Here's the drawing with two shaded views (mm, measured from the low corner). I have some questions. A direction names the side the tool comes from. Round coordinates to 2 decimals unless told otherwise and drop trailing zeros. Loops run counter-clockwise (first coordinate to the right, second up) from the corner with the lowest first, then second, coordinate; pieces in that order, holes last.
(1) Will these pins go through, and if not, where does the flat tip stop? pin 1 Ø1.5 at (y, z) = (26, 8.5) entering from -X; pin 2 Ø1.7 at (x, z) = (5, 12) entering from +Y; pin 3 Ø1 at (y, z) = (13.5, 3) entering from +X; pin 4 Ø5 at (x, y) = (16, 26) entering from -Z.
(2) Thinking about a two-plate mould opening in Z: for the marked faces 1, 2, 3 and 4, which applies, released by +Z, released by -Z, zero draft, split by the parting line, or undercut?
(3) Which directions (+Z, -Z, +X, -X, +Y, -Y) give clear straight access to the entire face, cutting with the end or side of a thin tool? Please do the marked faces 5, 6, 7, 8 and 9.
(4) I want a section at C-C on x = 16. Write out the boundary of the cut face in (y, z), plus the area to 3 significant figures.
(5) If I drill on line 1 along Y through (x, z) = (6.25, 8.75); line 2 along Z through (x, y) = (7, 13.25); line 3 along X through (y, z) = (4, 10.75), over which ranges is the centre line in solid material (lowest first)?
(6) I want a section at B-B on x = 5. Write out the boundary of the cut face in (y, z).
(7) I want a section at D-D on y = 26. Write out the boundary of the cut face in (x, z).
(8) I want a section at A-A on z = 4.5. Write out the boundary of the cut face in (x, y).
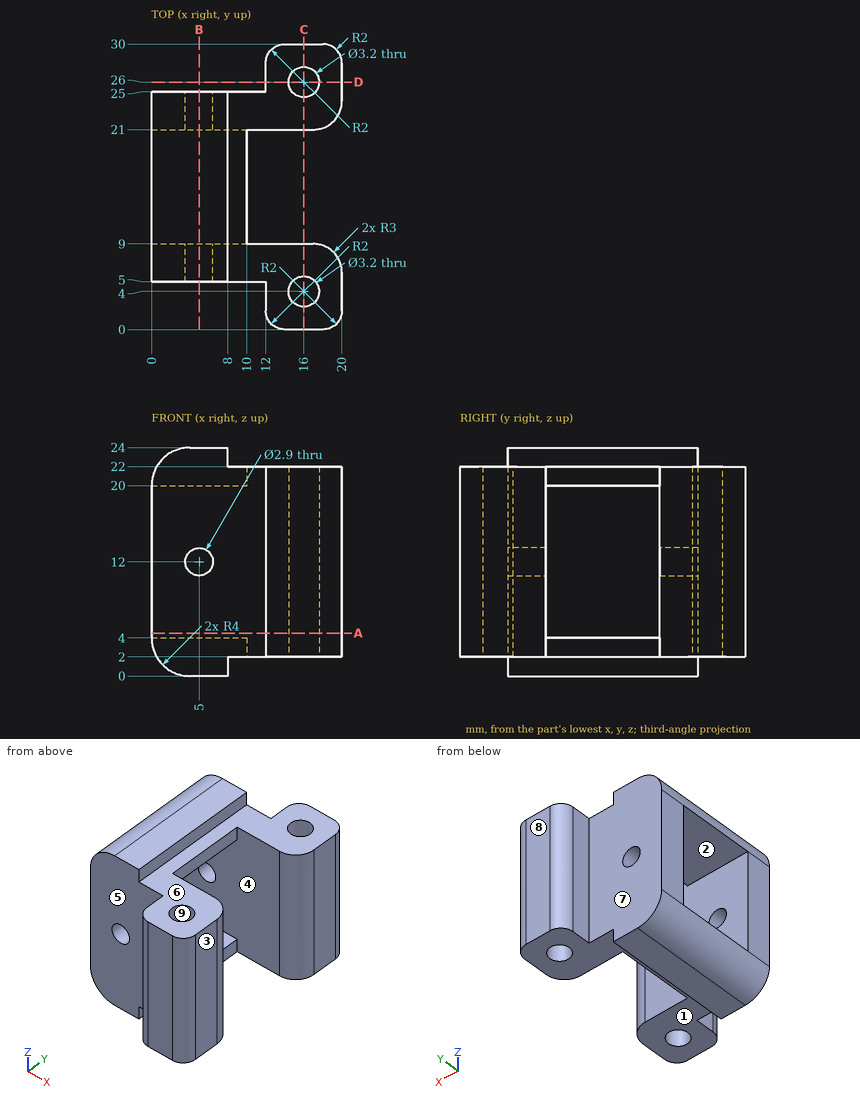
Filled sheet:
1. pin 1: stops at x = 12
1. pin 2: passes through
1. pin 3: stops at x = 10
1. pin 4: stops at z = 2
2. face 1: released by -Z
2. face 2: undercut
2. face 3: zero draft
2. face 4: undercut
3. face 5: +Z, -Z, -X, -Y
3. face 6: +Z, +X, +Y, -Y
3. face 7: +Z, -Z, -X, +Y
3. face 8: +Z, -Z, +X, -X, +Y
3. face 9: +Z, -Z
4. outline: (0, 2) - (2.4, 2) - (2.4, 22) - (0, 22) - close; (5.6, 2) - (9, 2) - (9, 22) - (5.6, 22) - close; (21, 2) - (24.4, 2) - (24.4, 22) - (21, 22) - close; (27.6, 2) - (30, 2) - (30, 22) - (27.6, 22) - close
4. area: 232 mm2
5. line 1: y = 5 to 9, 21 to 25
5. line 2: z = 0 to 4, 20 to 24
5. line 3: x = 12 to 14.4, 17.6 to 20
6. outline: (5, 0) - (25, 0) - (25, 10.55) - (21, 10.55) - (21, 4) - (9, 4) - (9, 10.55) - (5, 10.55) - close; (5, 13.45) - (9, 13.45) - (9, 20) - (21, 20) - (21, 13.45) - (25, 13.45) - (25, 24) - (5, 24) - close
7. outline: (12, 2) - (14.4, 2) - (14.4, 22) - (12, 22) - close; (17.6, 2) - (20, 2) - (20, 22) - (17.6, 22) - close
8. outline: (0, 5) - (12, 5) - (12, 2) arc R2 ccw to (14, 0) - (18, 0) arc R2 ccw to (20, 2) - (20, 6) arc R3 ccw to (17, 9) - (0, 9) - close; (0, 21) - (17, 21) arc R3 ccw to (20, 24) - (20, 28) arc R2 ccw to (18, 30) - (14, 30) arc R2 ccw to (12, 28) - (12, 25) - (0, 25) - close; hole circle Ø3.2 at (16, 4); hole circle Ø3.2 at (16, 26)
